Design review of the part built by this model. Coordinates are the model's own, in mm. A direction names the side the tool comes from. Round coordinates to 2 decimals unless told otherwise and drop trailing zeros. Loops run counter-clockwise (first coordinate to the right, second up) from the corner with the lowest first, then second, coordinate; pieces in that order, holes last. Notation, with made-up numbers: (76, 28.5) - (80, 28.5) arc R19 ccw to (80, 52.5) - close; hole circle Ø9 at (-11, 33). An arc over 180 degrees is marked (long way). Use one line per item in the form item = value. Start each with the question number.
(1) Machinability: for faces 1 (the cylindrical face through (7.1, 61.68, -3.69)), 2 (the cylindrical face through (1.532, 190.61, -3.695)), which of the approach directions +Z, -Z, +X, -X, +Y, -Y give a long, thin tool a straight path to every point of the face, cutting with its end or side? Answer none if there is none.
(2) Wall thickness on probe 1 along Z at (x, y) = (0.25, 64); probe 2 along Y at (x, z) = (-5.25, 1); probe 3 along X at (y, z) = (78, 0.5): over which ranges is each line inside the solid? List them lowest first. Write a range as [from, to].
(3) For pin 1 (6 mm diameter, centred on x = -5, y = 121, fed in from -Z); pin 2 (2 mm diameter, centred on x = -3, z = -2, fed in from -Y); pin 3 (1 mm diameter, centred on x = -3.5, y = 138, fed in from +Z); pin 4 (1 mm diameter, centred on y = 146.5, z = 6, fed in from -X), all flat-tipped, find the tip position at first contact; note any pin that passes through.
(4) We need section A-A, the plane y = 53. Write out the cut boundary in (x, z).
(5) We need section B-B, the plane y = 163.5. Write out the cut boundary in (x, z).
from build123d import *

# Parameters (mm, degrees)
FILLET1_R = 3
FILLET2_R = 3
FILLET3_R = 3
FILLET4_R = 6


with BuildPart() as part:
    # Sketch1 → Revolve1 (revolve)
    with BuildSketch(Plane.XY, mode=Mode.PRIVATE) as revolve1_sk:
        Polygon((0, 0), (0, 260), (-4, 260), (-4, 125), (-8, 120), (-8, 0), align=None)
    revolve(revolve1_sk.sketch.rotate(Axis((0, 0, 0), (0, 1, 0)), 270), axis=Axis((0, 0, 0), (0, 1, 0)))

    # Fillet1
    fillet1_edges = [part.edges().sort_by_distance(p)[0] for p in [
        (0, 260, 4),
    ]]
    fillet(fillet1_edges, radius=FILLET1_R)

    # Fillet2
    fillet2_edges = [part.edges().sort_by_distance(p)[0] for p in [
        (0, 120, 8),
    ]]
    fillet(fillet2_edges, radius=FILLET2_R)

    # Fillet3
    fillet3_edges = [part.edges().sort_by_distance(p)[0] for p in [
        (0, 125, 4),
    ]]
    fillet(fillet3_edges, radius=FILLET3_R)

    # Fillet4
    fillet4_edges = [part.edges().sort_by_distance(p)[0] for p in [
        (0, 0, 8),
    ]]
    fillet(fillet4_edges, radius=FILLET4_R)


solid = part.part
Data:
q1.face_1 = +Y, -Y
q1.face_2 = +Y
q2.probe_1 = [-8, 8]
q2.probe_2 = [1.02, 123.32]
q2.probe_3 = [-7.98, 7.98]
q3.pin_1 = -7.58
q3.pin_2 = 0.03
q3.pin_3 = 2.65
q3.pin_4 = through
q4.outline = circle Ø16 at (0, 0)
q5.outline = circle Ø8 at (0, 0)
